Design review of the part built by this model. Coordinates are the model's own, in mm. Face numbers are marked on the shaded views. A direction names the side the tool comes from. Coordinates: 2 decimals unless noted, no trailing zeros. Order: outer loops, then holes, each group sorted by start corner. A loop starts at its lowest first (then second) coordinate and runs counter-clockwise, first axis right, second up. Notation, with made-up numbers: (19.5, -1.75) -> (60.5, -1.75) arc R16 cw to (60.5, 29.25) -> close; hole circle Ø1 at (32.5, -32.5). An arc over 180 degrees is marked (long way). Write item = value, one per line.
```python
from build123d import *

# Parameters (mm, degrees)
PAD_DEPTH     = 20.2
SKETCH001_R   = 2.9
SKETCH001_R_2 = 1.5
POCKET_DEPTH  = 2


with BuildPart() as part:
    # Sketch → Pad (new body)
    with BuildSketch(Plane.XY):
        with BuildLine():
            Line((-27.8, 17.35), (-25.8, 17.35))
            Line((-25.8, 17.35), (-25.8, -17.35))
            Line((-25.8, -17.35), (25.8, -17.35))
            Line((25.8, -17.35), (25.8, 17.35))
            Line((25.8, 17.35), (27.8, 17.35))
            Line((27.8, 17.35), (27.8, -17.1))
            ThreePointArc((25.55, -19.35), (27.14099, -18.69099), (27.8, -17.1))
            Line((25.55, -19.35), (-25.55, -19.35))
            ThreePointArc((-27.8, -17.1), (-27.14099, -18.69099), (-25.55, -19.35))
            Line((-27.8, -17.1), (-27.8, 17.35))
        make_face()
    extrude(amount=PAD_DEPTH)

    # Sketch001 (on Face9 of Pad) → Pocket (cut)
    with BuildSketch(Plane.XZ.offset(19.35)):
        with Locations((0, 10.1)):
            Circle(SKETCH001_R)
        with Locations((5, 15.1)):
            Circle(SKETCH001_R_2)
        with Locations((-5, 15.1)):
            Circle(SKETCH001_R_2)
        with Locations((-5, 5.1)):
            Circle(SKETCH001_R_2)
        with Locations((5, 5.1)):
            Circle(SKETCH001_R_2)
        with Locations((-15, 15.1)):
            Circle(SKETCH001_R_2)
        with Locations((-15, 5.1)):
            Circle(SKETCH001_R_2)
        with Locations((15, 15.1)):
            Circle(SKETCH001_R_2)
        with Locations((15, 5.1)):
            Circle(SKETCH001_R_2)
    extrude(amount=-POCKET_DEPTH, mode=Mode.SUBTRACT)


solid = part.part
```
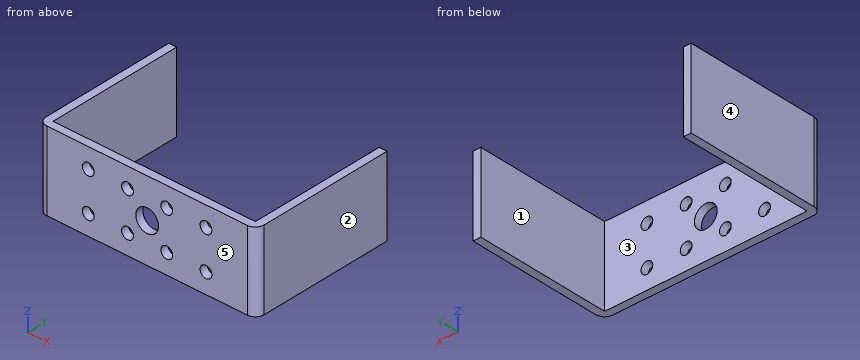
(1) We need section D-D (y = -14). Write out the cut boundary in (x, z), and give its area (3 significant figures).
Report:
outline = (-27.8, 0) -> (-25.8, 0) -> (-25.8, 20.2) -> (-27.8, 20.2) -> close; (25.8, 0) -> (27.8, 0) -> (27.8, 20.2) -> (25.8, 20.2) -> close
area = 80.8 mm²
(2) We need section C-C (x = 0). Write out the cut boundary in (y, z), and give its area (3 significant figures).
Report:
outline = (-19.35, 0) -> (-17.35, 0) -> (-17.35, 7.2) -> (-19.35, 7.2) -> close; (-19.35, 13) -> (-17.35, 13) -> (-17.35, 20.2) -> (-19.35, 20.2) -> close
area = 28.8 mm²
(3) For L1, parallel to Z at x = 15, y = -18; L2, parallel to X at y = -12, z = 1.5; L3, parallel to Y at x = -23, z = 13, list the stretches that pass through material, from the lowest coordinate up.
Report:
L1 = 0 to 3.6, 6.6 to 13.6, 16.6 to 20.2
L2 = -27.8 to -25.8, 25.8 to 27.8
L3 = -19.35 to -17.35
(4) We need section A-A (x = 15). Write out the cut boundary in (y, z).
Report:
outline = (-19.35, 0) -> (-17.35, 0) -> (-17.35, 3.6) -> (-19.35, 3.6) -> close; (-19.35, 6.6) -> (-17.35, 6.6) -> (-17.35, 13.6) -> (-19.35, 13.6) -> close; (-19.35, 16.6) -> (-17.35, 16.6) -> (-17.35, 20.2) -> (-19.35, 20.2) -> close
(5) Insertion check: pin 1 (1 mm diameter, centred on x = 12, z = 16, fed in from +Y). The pin has a flat end and moves straight along its axis. Give the tip position at first contact, or say it passes through.
Report:
pin_1 = -17.35
(6) We need section B-B (z = 10.1). Write out the cut boundary in (x, y).
Report:
outline = (-27.8, -17.1) arc R2.25 ccw to (-25.55, -19.35) -> (-2.9, -19.35) -> (-2.9, -17.35) -> (-25.8, -17.35) -> (-25.8, 17.35) -> (-27.8, 17.35) -> close; (2.9, -19.35) -> (25.55, -19.35) arc R2.25 ccw to (27.8, -17.1) -> (27.8, 17.35) -> (25.8, 17.35) -> (25.8, -17.35) -> (2.9, -17.35) -> close
(7) The part is to be moulded in two halves that separate along X. For the marked faces 3, 4 and 5, say which applies: released by +X, released by -X, zero draft, split by the parting line, or undercut.
Report:
face_3 = undercut
face_4 = released by -X
face_5 = zero draft
(8) For the marked faces 1 and 2, list the 3-axis set-ups (+Z, -Z, +X, -X, +Y, -Y) from which the entire face can be reached by the end or side of a thin tool; tool diameter is ignored.
Report:
face_1 = +Z, -Z, +Y
face_2 = +Z, -Z, +X, +Y, -Y
